from build123d import *

# Parameters (mm, degrees)
SKETCH1_R           = 12.7
BOSS_EXTRUDE1_DEPTH = 76.2
SKETCH2_R           = 6.35
BOSS_EXTRUDE2_DEPTH = 25.4


with BuildPart() as part:
    # Sketch1 → Boss-Extrude1 (new body)
    with BuildSketch(Plane.XY):
        Circle(SKETCH1_R)
        Polygon((2.54, 0), (2.54, 76.2), (-2.54, 76.2), (-2.54, 0), (-2.54, -76.2), (2.54, -76.2), align=None)
        Polygon((1.27, -2.199704526), (67.261135768, 35.900295474), (64.721135768, 40.299704526), (-1.27, 2.199704526), (-67.261135768, -35.900295474), (-64.721135768, -40.299704526), align=None)
        Polygon((-1.27, -2.199704526), (64.721135768, -40.299704526), (67.261135768, -35.900295474), (1.27, 2.199704526), (-64.721135768, 40.299704526), (-67.261135768, 35.900295474), align=None)
    extrude(amount=BOSS_EXTRUDE1_DEPTH)

    # Sketch2 → Boss-Extrude2 (add)
    with BuildSketch(Plane.XY.offset(76.2)):
        Circle(SKETCH2_R)
    extrude(amount=BOSS_EXTRUDE2_DEPTH)


solid = part.part
Verification items for the finished model (mm, model axes). A direction names the side the tool comes from. Round coordinates to 2 decimals unless told otherwise and drop trailing zeros. Order: outer loops, then holes, each group sorted by start corner. A loop starts at its lowest first (then second) coordinate and runs counter-clockwise, first axis right, second up. Notation, with made-up numbers: (2, 85.5) -> (54, 85.5) arc R4 ccw to (54, 90.5) -> close; hole circle Ø3 at (9, -35). An arc over 180 degrees is marked (long way). Put each result on its own line as item: value.
1) Section check A-A (y = -18.5). Record the cut outline in (x, z), then the cut area to 3 significant figures.
Final values:
outline: (-37.12, 0) -> (-26.96, 0) -> (-26.96, 76.2) -> (-37.12, 76.2) -> close; (-2.54, 0) -> (2.54, 0) -> (2.54, 76.2) -> (-2.54, 76.2) -> close; (26.96, 0) -> (37.12, 0) -> (37.12, 76.2) -> (26.96, 76.2) -> close
area: 1,940 mm^2
2) Set-up check for faces 1 (the flat face through (-39.27, -19.74, 37.57)), 2 (the flat face through (39.27, 19.74, 37.57)), 3 (the flat face through (-2.54, -44, 38)): record each of +Z, -Z, +X, -X, +Y, -Y from which the full face is reachable in a straight line by a thin tool's end or side.
Final values:
face 1: +Z, -Z, -X
face 2: +Z, -Z, +X
face 3: +Z, -Z, -Y
3) Section check D-D (x = 0). Record the cut outline in (y, z).
Final values:
outline: (-76.2, 0) -> (76.2, 0) -> (76.2, 76.2) -> (6.35, 76.2) -> (6.35, 101.6) -> (-6.35, 101.6) -> (-6.35, 76.2) -> (-76.2, 76.2) -> close
4) Material ranges on line 1 (X direction, y = -32.5, z = 46.5); line 2 (X direction, y = 23.5, z = 66); line 3 (Y direction, x = 4, z = 66), recorded low to high.
Final values:
line 1: x = -61.37 to -51.21, -2.54 to 2.54, 51.21 to 61.37
line 2: x = -45.78 to -35.62, -2.54 to 2.54, 35.62 to 45.78
line 3: y = -12.05 to 12.05
5) Depth check by flat-ended pin: pin 1 (2 mm diameter, centred on y = 33, z = 64, fed in from +X); pin 2 (6 mm diameter, centred on y = -38, z = 73, fed in from +X); pin 3 (1 mm diameter, centred on x = -48, z = 50.5, fed in from -Y); pin 4 (10 mm diameter, centred on x = 51.5, y = 30, fed in from -Z). Enter the tip coordinate at first touch or a pass-through.
Final values:
pin 1: stops at x = 63.97
pin 2: stops at x = 67.26
pin 3: stops at y = -30.93
pin 4: stops at z = 0
6) Section check B-B (z = 22). Record the cut outline in (x, y).
Final values:
outline: (-67.26, -35.9) -> (-64.72, -40.3) -> (-9.51, -8.42) arc R12.7 ccw to (-2.54, -12.44) -> (-2.54, -76.2) -> (2.54, -76.2) -> (2.54, -12.44) arc R12.7 ccw to (9.51, -8.42) -> (64.72, -40.3) -> (67.26, -35.9) -> (12.05, -4.02) arc R12.7 ccw to (12.05, 4.02) -> (67.26, 35.9) -> (64.72, 40.3) -> (9.51, 8.42) arc R12.7 ccw to (2.54, 12.44) -> (2.54, 76.2) -> (-2.54, 76.2) -> (-2.54, 12.44) arc R12.7 ccw to (-9.51, 8.42) -> (-64.72, 40.3) -> (-67.26, 35.9) -> (-12.05, 4.02) arc R12.7 ccw to (-12.05, -4.02) -> close
7) Mould release check, pull along Z, two halves, no side actions. Record for faces 4 (the flat face through (0, 0, 0)), 5 (the cylindrical face through (-12.7, 0.1, 37.6)), 6 (the flat face through (5, -5, 76.2)): +Z half, -Z half, draft (parallel to the pull), parting line (faces both ways), or undercut.
Final values:
face 4: -Z half
face 5: draft
face 6: +Z half
8) Section check C-C (x = -42). Record the cut outline in (y, z).
Final values:
outline: (-27.18, 0) -> (-21.32, 0) -> (-21.32, 76.2) -> (-27.18, 76.2) -> close; (21.32, 0) -> (27.18, 0) -> (27.18, 76.2) -> (21.32, 76.2) -> close
